```python
from build123d import *

# Parameters (mm, degrees)
M6X1_0_TAPPED_HOLE1_D     = 5
M6X1_0_TAPPED_HOLE1_DEPTH = 7
M6X1_0_TAPPED_HOLE1_TIP   = 1.502151548


with BuildPart() as part:
    # Sketch1 → Revolve1 (revolve)
    with BuildSketch(Plane.XY, mode=Mode.PRIVATE) as revolve1_sk:
        Polygon((0, 0), (5.5, 0), (5.5, 31.5), (7, 31.5), (7.5, 32), (7.5, 52), (7, 52.5), (5.5, 52.5), (5.5, 95.5), (0, 95.5), align=None)
    revolve(revolve1_sk.sketch.rotate(Axis((0, 0, 0), (0, 1, 0)), 90), axis=Axis((0, 0, 0), (0, 1, 0)))

    # M6x1.0 Tapped Hole1
    with Locations(Plane(origin=(0, 0, 0), x_dir=(-1, 0, 0), z_dir=(0, -1, 0))):
        with Locations((0, 0)):
            Hole(M6X1_0_TAPPED_HOLE1_D / 2, depth=M6X1_0_TAPPED_HOLE1_DEPTH)
            with Locations((0, 0, -(M6X1_0_TAPPED_HOLE1_DEPTH + M6X1_0_TAPPED_HOLE1_TIP / 2))):  # 118° drill point
                Cone(0, M6X1_0_TAPPED_HOLE1_D / 2, M6X1_0_TAPPED_HOLE1_TIP, mode=Mode.SUBTRACT)


solid = part.part
```
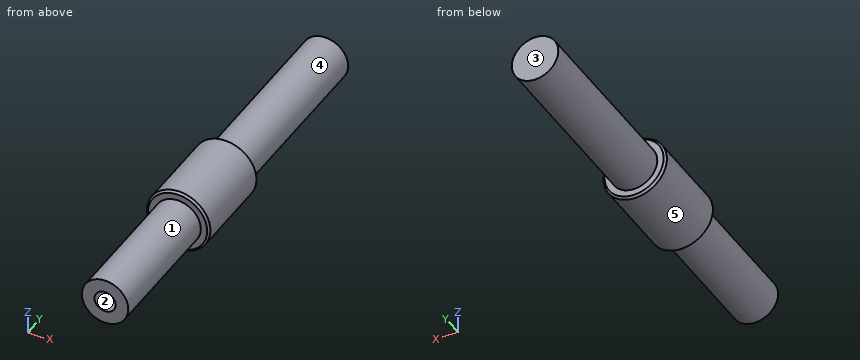
For this review, take the finished solid that the model builds, in its own axes (mm). Face numbers are marked on the shaded views. A direction names the side the tool comes from. Round coordinates to 2 decimals unless told otherwise and drop trailing zeros. Write each loop counter-clockwise with the first axis right and the second up, starting at its lowest first coordinate (ties: lowest second). Pieces come first, ordered by that corner, then holes.
1) Insertion check: pin 1 Ø4 at (x, y) = (6, 65.5) entering from +Z; pin 2 Ø1.5 at (x, y) = (-4, 22.5) entering from +Z; pin 3 Ø1 at (y, z) = (71.5, -3.5) entering from +X; pin 4 Ø8 at (x, z) = (0, 0) entering from -Y. Each pin has a flat end and moves straight along its axis. Give the tip position at first contact, or say it passes through.
Answer below:
pin 1: stops at z = 3.77
pin 2: stops at z = 4.44
pin 3: stops at x = 4.61
pin 4: stops at y = 0
2) Take a section at A-A on y = 50. Give the boundary of the cut face in (x, z).
Answer below:
outline: circle Ø15 at (0, 0)
3) For line 1 along Y through (x, z) = (-6, 0); line 2 along Y through (x, z) = (-0.75, 1.5); line 3 along X through (y, z) = (40, 4.5), list the stretches that pass through material, from the lowest coordinate up.
Answer below:
line 1: y = 31.5 to 52.5
line 2: y = 7.49 to 95.5
line 3: x = -6 to 6
4) Take a section at B-B on y = 86. Give the boundary of the cut face in (x, z).
Answer below:
outline: circle Ø11 at (0, 0)
5) Machinability: for the marked faces 4 and 5, which of the approach directions +Z, -Z, +X, -X, +Y, -Y give a long, thin tool a straight path to every point of the face, cutting with its end or side? Answer none if there is none.
Answer below:
face 4: +Y
face 5: +Y, -Y
6) Mouldability with a two-part tool opening along X and no side actions: class the marked faces 1, 2 and 3 as +X half, -X half, draft (parallel to the pull), parting line (faces both ways), or undercut.
Answer below:
face 1: parting line
face 2: undercut
face 3: draft
